Here's how the part is built. I have some questions about the finished solid (model axes, mm). Face numbers are marked on the shaded views. A direction names the side the tool comes from. Coordinates: 2 decimals unless noted, no trailing zeros. Loops run counter-clockwise (first coordinate to the right, second up) from the corner with the lowest first, then second, coordinate; pieces in that order, holes last.
from build123d import *

# Parameters (mm, degrees)
EXTRUDE_1_DEPTH     = 60
SKETCH_2_R          = 4
SKETCH_2_R_2        = 2.1
CUT_EXTRUDE_1_DEPTH = 36
SKETCH_3_R          = 0.2
CUT_EXTRUDE_2_DEPTH = 70
FILLET_1_R          = 0.5


with BuildPart() as part:
    # 草图1 → 凸台-拉伸1 (new body)
    with BuildSketch(Plane.XY):
        Polygon((0, 0), (19, 0), (19, 32), (57, 32), (57, 35), (16, 35), (16, 3), (0, 3), align=None)
    extrude(amount=EXTRUDE_1_DEPTH)

    # 草图2 → 切除-拉伸1 (cut, through all)
    with BuildSketch(Plane(origin=(0, 35, 0), x_dir=(1, 0, 0), z_dir=(0, 1, 0))):
        with Locations((45, -30)):
            Circle(SKETCH_2_R)
        with Locations((10, -30)):
            Circle(SKETCH_2_R_2)
        with Locations((10, -50)):
            Circle(SKETCH_2_R_2)
        with Locations((10, -10)):
            Circle(SKETCH_2_R_2)
    extrude(amount=-CUT_EXTRUDE_1_DEPTH, mode=Mode.SUBTRACT)

    # 草图3 → 切除-拉伸2 (cut)
    with BuildSketch(Plane.XY.offset(60)):
        with Locations((10, 0)):
            Circle(SKETCH_3_R)
        with Locations((45, 35)):
            Circle(SKETCH_3_R)
    extrude(amount=-CUT_EXTRUDE_2_DEPTH, mode=Mode.SUBTRACT)

    # 圆角1
    fillet_1_edges = [part.edges().sort_by_distance(p)[0] for p in [
        (0, 3, 30),
        (16, 35, 30),
        (57, 35, 30),
        (57, 32, 30),
        (19, 0, 30),
        (0, 0, 30),
    ]]
    fillet(fillet_1_edges, radius=FILLET_1_R)


solid = part.part
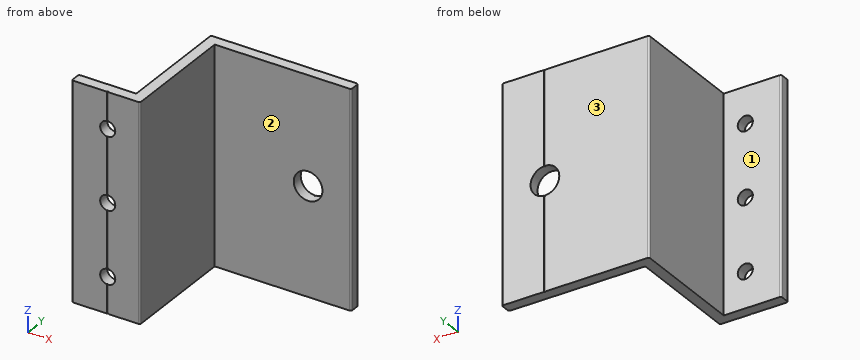
Q1. For the marked faces 1, 2 and 3, which set-ups out of +Z, -Z, +X, -X, +Y, -Y let a thin tool reach every point of the face, with its end or its side?
Q2. Please list where these lines run through material, in increasing order: probe 1 along Z at (x, y) = (10, 1); probe 2 along X at (y, z) = (0.95, 50); probe 3 along Z at (x, y) = (45, 33.4).
Q3. Suppose I cut it at B-B on z = 10. Write out the boundary of the cut face in (x, y).
Q4. Suppose I cut it at D-D on z = 16.5. Write out the boundary of the cut face in (x, y), and give its area (3 significant figures).
Q5. Will these pins go through, and if not, where does the flat tip stop? P1, Ø10.5, axis at x = 45, z = 30, coming from the -Y side; P2, Ø4, axis at x = 10, z = 30, coming from the +Y side (3 decimals); P3, Ø8, axis at x = 11.5, z = 30, coming from the +Y side; P4, Ø5, axis at y = 8.5, z = 36, coming from the -X side.
Q6. Suppose I cut it at C-C on y = 9. Write out the boundary of the cut face in (x, z).
Q7. Suppose I cut it at A-A on z = 30. Write out the boundary of the cut face in (x, y).
Check values:
1. face 1: +Z, -Z, -X, +Y
1. face 2: +Z, -Z, +X, -Y
1. face 3: +Z, -Z, +X, -X, +Y
2. probe 1: z = 0 to 7.9, 12.1 to 27.9, 32.1 to 47.9, 52.1 to 60
2. probe 2: x = 0 to 7.9, 12.1 to 19
2. probe 3: z = 0 to 26, 34 to 60
3. outline: (0, 0.5) arc R0.5 ccw to (0.5, 0) - (7.9, 0) - (7.9, 3) - (0.5, 3) arc R0.5 ccw to (0, 2.5) - close; (12.1, 0) - (18.5, 0) arc R0.5 ccw to (19, 0.5) - (19, 32) - (56.5, 32) arc R0.5 ccw to (57, 32.5) - (57, 34.5) arc R0.5 ccw to (56.5, 35) - (45.2, 35) arc R0.2 cw to (44.8, 35) - (16.5, 35) arc R0.5 ccw to (16, 34.5) - (16, 3) - (12.1, 3) - close
4. outline: (0, 0.5) arc R0.5 ccw to (0.5, 0) - (9.8, 0) arc R0.2 cw to (10.2, 0) - (18.5, 0) arc R0.5 ccw to (19, 0.5) - (19, 32) - (56.5, 32) arc R0.5 ccw to (57, 32.5) - (57, 34.5) arc R0.5 ccw to (56.5, 35) - (45.2, 35) arc R0.2 cw to (44.8, 35) - (16.5, 35) arc R0.5 ccw to (16, 34.5) - (16, 3) - (0.5, 3) arc R0.5 ccw to (0, 2.5) - close
4. area: 267 mm2
5. P1: stops at y = 32
5. P2: passes through
5. P3: stops at y = 3
5. P4: stops at x = 16
6. outline: (16, 0) - (19, 0) - (19, 60) - (16, 60) - close
7. outline: (0, 0.5) arc R0.5 ccw to (0.5, 0) - (7.9, 0) - (7.9, 3) - (0.5, 3) arc R0.5 ccw to (0, 2.5) - close; (12.1, 0) - (18.5, 0) arc R0.5 ccw to (19, 0.5) - (19, 32) - (41, 32) - (41, 35) - (16.5, 35) arc R0.5 ccw to (16, 34.5) - (16, 3) - (12.1, 3) - close; (49, 32) - (56.5, 32) arc R0.5 ccw to (57, 32.5) - (57, 34.5) arc R0.5 ccw to (56.5, 35) - (49, 35) - close
